```python
from build123d import *

# Parameters (mm, degrees)
BOSS_EXTRUDE2_DEPTH      = 8.5
BOSS_EXTRUDE2_DEPTH_BACK = 8.5
SKETCH1_R                = 6
CUT_EXTRUDE1_DEPTH       = 5.5
CUT_EXTRUDE1_DEPTH_BACK  = 5.5
SKETCH1_4_R              = 6
CUT_EXTRUDE2_DEPTH       = 68.492341935
CUT_EXTRUDE2_DEPTH_BACK  = 68.492341935
SKETCH3_R                = 3
SKETCH3_3_R              = 7
SKETCH3_3_R_2            = 3
CUT_EXTRUDE3_DEPTH       = 6
CUT_EXTRUDE4_DEPTH       = 10


with BuildPart() as part:
    # Sketch1 → Boss-Extrude2 (new, two sides: drawn at the far end of the back side and taken through both)
    # profile 1 of 3: a face of its own
    with BuildSketch(Plane(origin=(0, 0, 0), x_dir=(0, 0, -1), z_dir=(1, 0, 0)).offset(-BOSS_EXTRUDE2_DEPTH_BACK)):
        Polygon((28, 0), (28, -7.65385), (28, -22.65385), (31, -22.65385), (31, -27.65385), (28, -27.65385), (28, -31.65385), (3, -31.65385), (3, 3), (-3, 3), (-3, -31.65385), (-28, -31.65385), (-28, -27.65385), (-31, -27.65385), (-31, -22.65385), (-28, -22.65385), (-28, -7.65385), (-28, 0), (-28, 18), (28, 18), align=None)
        Polygon((-24.5, -24.850002423), (-15.5, -30.046154845), (-6.5, -24.850002423), (-6.5, -14.457697577), (-15.5, -9.261545155), (-24.5, -14.457697577), align=None, mode=Mode.SUBTRACT)
        Polygon((6.5, -24.850002423), (15.5, -30.046154845), (24.5, -24.850002423), (24.5, -14.457697577), (15.5, -9.261545155), (6.5, -14.457697577), align=None, mode=Mode.SUBTRACT)
    # profile 2 of 3: a face of its own
    with BuildSketch(Plane(origin=(0, 0, 0), x_dir=(0, 0, -1), z_dir=(1, 0, 0)).offset(-BOSS_EXTRUDE2_DEPTH_BACK)):
        Polygon((-24.5, -14.457697577), (-24.5, -24.850002423), (-15.5, -30.046154845), (-6.5, -24.850002423), (-6.5, -14.457697577), (-15.5, -9.261545155), align=None)
        with Locations((-15.5, -19.65385)):
            Circle(SKETCH1_R, mode=Mode.SUBTRACT)
    # profile 3 of 3: a face of its own
    with BuildSketch(Plane(origin=(0, 0, 0), x_dir=(0, 0, -1), z_dir=(1, 0, 0)).offset(-BOSS_EXTRUDE2_DEPTH_BACK)):
        Polygon((6.5, -14.457697577), (6.5, -24.850002423), (15.5, -30.046154845), (24.5, -24.850002423), (24.5, -14.457697577), (15.5, -9.261545155), align=None)
        with Locations((15.5, -19.65385)):
            Circle(SKETCH1_R, mode=Mode.SUBTRACT)
    extrude(amount=BOSS_EXTRUDE2_DEPTH + BOSS_EXTRUDE2_DEPTH_BACK)

    # Sketch1_4 → Cut-Extrude1 (cut, two sides: drawn at the far end of the back side and taken through both)
    # profile 1 of 2: a face of its own
    with BuildSketch(Plane(origin=(0, 0, 0), x_dir=(0, 0, -1), z_dir=(1, 0, 0)).offset(-CUT_EXTRUDE1_DEPTH_BACK)):
        Polygon((-24.5, -31.65385), (-6.5, -31.65385), (-6.5, -14.457697577), (-15.5, -9.261545155), (-24.5, -14.457697577), align=None)
        with Locations((-15.5, -19.65385)):
            Circle(SKETCH1_4_R, mode=Mode.SUBTRACT)
    # profile 2 of 2: a face of its own
    with BuildSketch(Plane(origin=(0, 0, 0), x_dir=(0, 0, -1), z_dir=(1, 0, 0)).offset(-CUT_EXTRUDE1_DEPTH_BACK)):
        Polygon((6.5, -31.65385), (24.5, -31.65385), (24.5, -14.457697577), (15.5, -9.261545155), (6.5, -14.457697577), align=None)
        with Locations((15.5, -19.65385)):
            Circle(SKETCH1_4_R, mode=Mode.SUBTRACT)
    extrude(amount=CUT_EXTRUDE1_DEPTH + CUT_EXTRUDE1_DEPTH_BACK, mode=Mode.SUBTRACT)

    # Sketch3 → Cut-Extrude2 (cut, two sides: drawn at the far end of the back side and taken through both)
    with BuildSketch(Plane.XY.offset(28).offset(-CUT_EXTRUDE2_DEPTH_BACK)):
        with Locations(Location((0, -5, 0), (0, 0, 90))):
            Circle(SKETCH3_R)
    extrude(amount=CUT_EXTRUDE2_DEPTH + CUT_EXTRUDE2_DEPTH_BACK, mode=Mode.SUBTRACT)

    # Sketch3_3 → Cut-Extrude3 (cut)
    with BuildSketch(Plane.XY.offset(28)):
        with Locations((0, -5)):
            Circle(SKETCH3_3_R)
        with Locations((0, -5)):
            Circle(SKETCH3_3_R_2, mode=Mode.SUBTRACT)
    extrude(amount=-CUT_EXTRUDE3_DEPTH, mode=Mode.SUBTRACT)

    # Sketch4 → Cut-Extrude4 (cut)
    with BuildSketch(Plane(origin=(0, 0, -28), x_dir=(-1, 0, 0), z_dir=(0, 0, -1))):
        Polygon((5.773502692, -5), (2.886751346, 0), (-2.886751346, 0), (-5.773502692, -5), (-2.886751346, -10), (2.886751346, -10), align=None)
    extrude(amount=-CUT_EXTRUDE4_DEPTH, mode=Mode.SUBTRACT)


solid = part.part
```
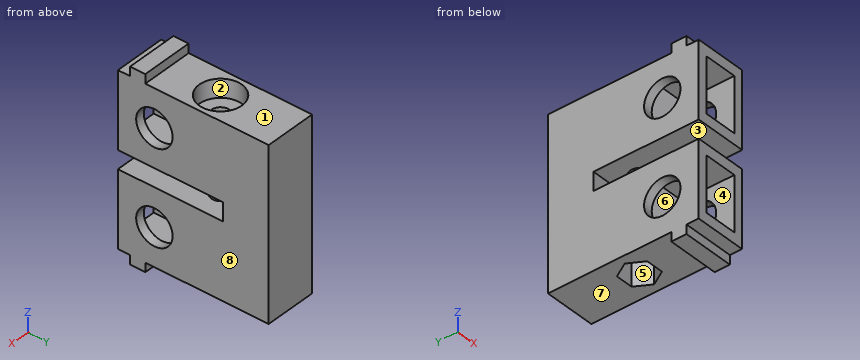
Can you work these out from the model? Positions are in its coordinate system, mm. Face numbers are marked on the shaded views. A direction names the side the tool comes from. Give positions to 0.01 mm unless a question says otherwise; leave off trailing zeros. Loops run counter-clockwise (first coordinate to the right, second up) from the corner with the lowest first, then second, coordinate; pieces in that order, holes last. Notation, with made-up numbers: M 32.5,77.25 L 44.5,77.25 A28 ccw 44.5,95.25 Z; hole C -7.75,66.25 d6. An arc over 180 degrees is marked long. Use one line per item in the form item = value. Start each with the question number.
(1) I want a section at D-D, the plane z = 0.5. Write out the boundary of the cut face in (x, y).
(2) Thinking about a two-plate mould opening in X: for the marked faces 6, 7 and 8, which applies, released by +X, released by -X, zero draft, split by the parting line, or undercut?
(3) On a 3-axis mill with a long thin cutter (end or side, diameter ignored), from which of +Z, -Z, +X, -X, +Y, -Y can I reach the whole of each face in a straight line? I mean the marked faces 1, 2, 3, 4 and 5. Say none if no direction works.
(4) I want a section at B-B, the plane y = -19. State how many separate pieces and enclosed holes the cut face has, and give its area (3 significant figures).
(5) I'm going to push flat-ended pins straight in: P1, Ø0.9, axis at x = 1, z = 30, coming from the -Y side; P2, Ø10, axis at x = 0, z = -19, coming from the -Y side; P3, Ø1.5, axis at x = 4.5, y = 11, coming from the -Z side. Where does each tip first touch, or does it pass through?
(6) Please list where these lines run through material, in increasing order: line 1 (Z direction, x = 5, y = -24.5); line 2 (Z direction, x = 0.5, y = -22); line 3 (Y direction, x = -6.75, z = 15.5).
(7) I want a section at A-A, the plane z = -11. Write out the boundary of the cut face in (x, y), and give its area (3 significant figures).
Worked out:
q1.outline = M -8.5,3 L 8.5,3 L 8.5,18 L -8.5,18 Z
q2.face_6 = undercut
q2.face_7 = zero draft
q2.face_8 = released by +X
q3.face_1 = +Z, +X, -X, +Y
q3.face_2 = +Z
q3.face_3 = +X, -X, -Y
q3.face_4 = -Y
q3.face_5 = -Z
q4.separate_pieces = 4
q4.enclosed_holes = 0
q4.area = 311 mm²
q5.P1 = -27.65
q5.P2 = -14.17
q5.P3 = -28
q6.line_1 = -31 to -24.5, -6.5 to -3, 3 to 6.5, 24.5 to 31
q6.line_2 = -28 to -24.5, -6.5 to -3, 3 to 6.5, 24.5 to 28
q6.line_3 = -31.65 to -25.65, -13.65 to 18
q7.outline = M -8.5,-31.65 L -5.5,-31.65 L -5.5,-23.62 L -8.5,-23.62 Z; M -8.5,-15.69 L -5.5,-15.69 L -5.5,-11.86 L 5.5,-11.86 L 5.5,-15.69 L 8.5,-15.69 L 8.5,18 L -8.5,18 Z; M 5.5,-31.65 L 8.5,-31.65 L 8.5,-23.62 L 5.5,-23.62 Z; hole C 0,-5 d6
q7.area = 550 mm²
